from build123d import *

# Parameters (mm, degrees)
SKETCH1_R           = 9
BOSS_EXTRUDE1_DEPTH = 65
SKETCH2_R           = 8
CUT_EXTRUDE1_DEPTH  = 0.2
SKETCH3_R           = 8
CUT_EXTRUDE2_DEPTH  = 0.2


with BuildPart() as part:
    # Sketch1 → Boss-Extrude1 (new body)
    with BuildSketch(Plane(origin=(0, 0, 0), x_dir=(1, 0, 0), z_dir=(0, 1, 0))):
        Circle(SKETCH1_R)
    extrude(amount=BOSS_EXTRUDE1_DEPTH)

    # Sketch2 → Cut-Extrude1 (cut)
    with BuildSketch(Plane(origin=(0, 65, 0), x_dir=(1, 0, 0), z_dir=(0, 1, 0))):
        Circle(SKETCH2_R)
    extrude(amount=-CUT_EXTRUDE1_DEPTH, mode=Mode.SUBTRACT)

    # Sketch3 → Cut-Extrude2 (cut)
    with BuildSketch(Plane.XZ):
        Circle(SKETCH3_R)
    extrude(amount=-CUT_EXTRUDE2_DEPTH, mode=Mode.SUBTRACT)


solid = part.part
The listing builds one solid part. Answer for the finished solid, in the listing's coordinates (mm). Give positions to 0.01 mm unless a question says otherwise; leave off trailing zeros. Write each loop counter-clockwise with the first axis right and the second up, starting at its lowest first coordinate (ties: lowest second). Pieces come first, ordered by that corner, then holes.
1) Given P1, Ø1.5, axis at y = 18.5, z = -2, coming from the +X side; P2, Ø1, axis at x = -1.5, y = 20, coming from the -Z side; P3, Ø6, axis at y = 33.5, z = -5, coming from the +X side, each flat-ended and moving along its own axis, determine where each tip first touches the part or whether it passes through.
2) For a pull along X with two mould halves and no side action, classify faces 1 (the face through (-1.172, 32.045, -8.923)), 2 (the face through (0, 0.2, 0)) as pulls with the +X half, pulls with the -X half, needs draft (parallel to the pull), parting line crosses it, or undercut.
3) Section B-B (y = 5) is taken. Write down the section's boundary in (x, z), and give its area (3 significant figures).
4) Section C-C (x = -6) is taken. Write down the section's boundary in (y, z).
5) Find the intervals of material crossed by L1, parallel to Z at x = 0, y = 64.9; L2, parallel to Y at x = -0.5, z = 5.75, in increasing order.
6) Section A-A (z = 2.75) is taken. Write down the section's boundary in (x, y).
Response:
1. P1: stops at x = 8.91
1. P2: stops at z = -8.94
1. P3: stops at x = 8.77
2. face 1: parting line crosses it
2. face 2: undercut
3. outline: circle Ø18 at (0, 0)
3. area: 254 mm2
4. outline: (0, -6.71) - (65, -6.71) - (65, -5.29) - (64.8, -5.29) - (64.8, 5.29) - (65, 5.29) - (65, 6.71) - (0, 6.71) - (0, 5.29) - (0.2, 5.29) - (0.2, -5.29) - (0, -5.29) - close
5. L1: z = -9 to -8, 8 to 9
5. L2: y = 0.2 to 64.8
6. outline: (-8.57, 0) - (-7.51, 0) - (-7.51, 0.2) - (7.51, 0.2) - (7.51, 0) - (8.57, 0) - (8.57, 65) - (7.51, 65) - (7.51, 64.8) - (-7.51, 64.8) - (-7.51, 65) - (-8.57, 65) - close
